```python
from build123d import *

# Parameters (mm, degrees)
BOSS_EXTRUDE1_DEPTH = 152.4
FILLET1_R           = 9.525


with BuildPart() as part:
    # Sketch2 → Boss-Extrude1 (new body, symmetric)
    with BuildSketch(Plane.XY):
        Polygon((-3.6195, 90.551), (-3.6195, -90.551), (-101.5365, -90.551), (-101.5365, -101.6), (101.5365, -101.6), (101.5365, -90.551), (3.6195, -90.551), (3.6195, 90.551), (101.5365, 90.551), (101.5365, 101.6), (-101.5365, 101.6), (-101.5365, 90.551), align=None)
    extrude(amount=BOSS_EXTRUDE1_DEPTH, both=True)

    # Fillet1
    fillet1_edges = [part.edges().sort_by_distance(p)[0] for p in [
        (-3.6195, -90.551, 0),
        (-3.6195, 90.551, 0),
        (3.6195, 90.551, 0),
        (3.6195, -90.551, 0),
    ]]
    fillet(fillet1_edges, radius=FILLET1_R)


solid = part.part
```
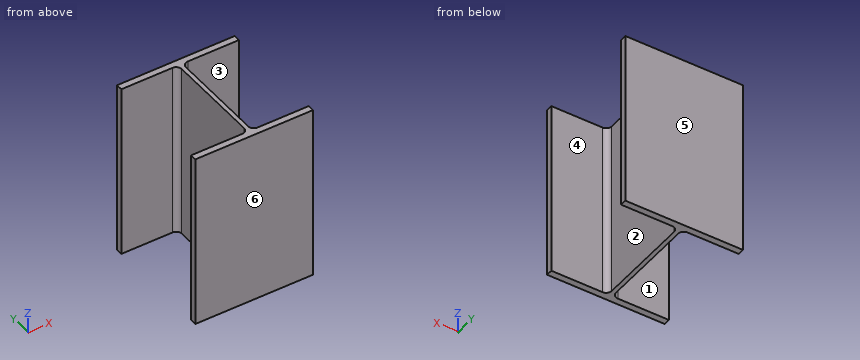
Verification items for the finished model (mm, model axes). Face numbers are marked on the shaded views. A direction names the side the tool comes from. Round coordinates to 2 decimals unless told otherwise and drop trailing zeros. Order: outer loops, then holes, each group sorted by start corner. A loop starts at its lowest first (then second) coordinate and runs counter-clockwise, first axis right, second up.
1) Tool access check on the marked faces 1 and 2. Record the directions out of +Z, -Z, +X, -X, +Y, -Y that give a thin tool (end or side, any length) a straight path to the whole face; none if there is none.
Geometry says:
face 1: +Z, -Z, -X
face 2: +Z, -Z, +X
2) Depth check by flat-ended pin: pin 1 (1 mm diameter, centred on y = -1.5, z = 93, fed in from +X); pin 2 (1.5 mm diameter, centred on y = 49, z = -17.5, fed in from -X). Enter the tip coordinate at first touch or a pass-through.
Geometry says:
pin 1: stops at x = 3.62
pin 2: stops at x = -3.62
3) Draft check along Y on the marked faces 3, 4, 5 and 6. Enter one of: +Y half, -Y half, draft (parallel to the pull), parting line (faces both ways), or undercut.
Geometry says:
face 3: undercut
face 4: undercut
face 5: +Y half
face 6: -Y half
4) Cross-section at A-A, the plane x = 45. Record the cut outline in (y, z), plus the area to 3 significant figures.
Geometry says:
outline: (-101.6, -152.4) - (-90.55, -152.4) - (-90.55, 152.4) - (-101.6, 152.4) - close; (90.55, -152.4) - (101.6, -152.4) - (101.6, 152.4) - (90.55, 152.4) - close
area: 6,740 mm2
5) Material ranges on line 1 (Y direction, x = 47.5, z = 66); line 2 (X direction, y = -35, z = 134.5); line 3 (Y direction, x = 10, z = -89), recorded low to high.
Geometry says:
line 1: y = -101.6 to -90.55, 90.55 to 101.6
line 2: x = -3.62 to 3.62
line 3: y = -101.6 to -90.02, 90.02 to 101.6
6) Cross-section at C-C, the plane y = 69.5. Record the cut outline in (x, z).
Geometry says:
outline: (-3.62, -152.4) - (3.62, -152.4) - (3.62, 152.4) - (-3.62, 152.4) - close
